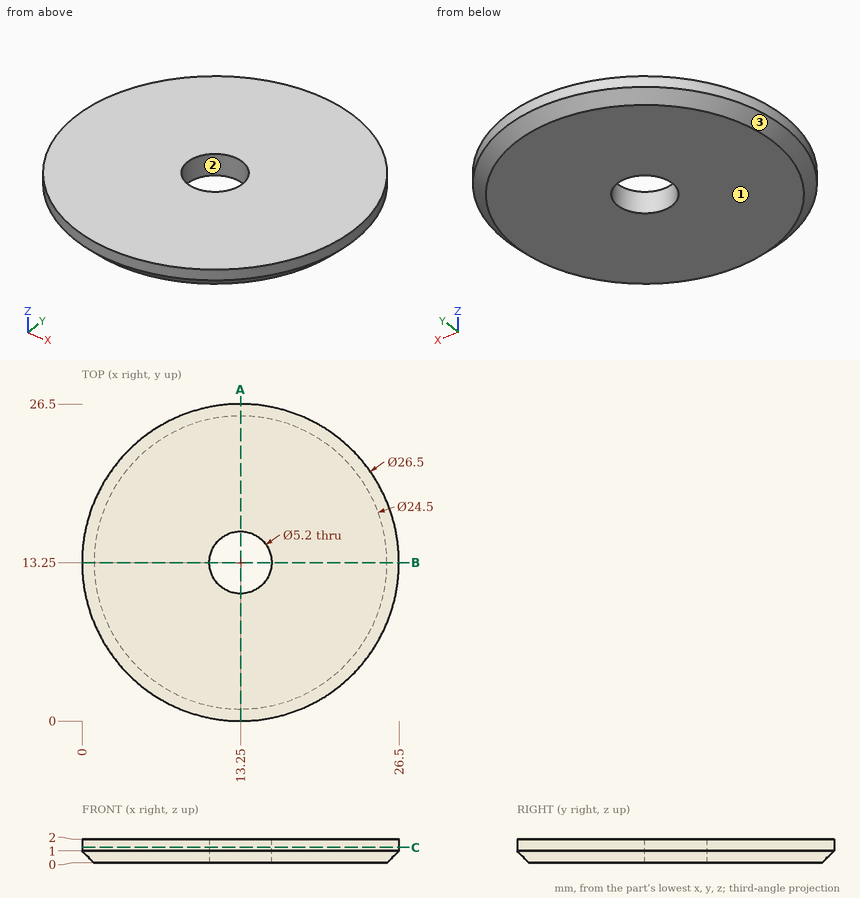
Study the drawing (mm; zero at the part's minimum x, y, z) and answer. Give positions to 0.01 mm unless a question says otherwise; leave off trailing zeros. Order: outer loops, then holes, each group sorted by start corner. A loop starts at its lowest first (then second) coordinate and runs counter-clockwise, first axis right, second up. Notation, with made-up numbers: (-25.75, -11) - (22.25, -11) arc R12 ccw to (22.25, 11) - close; hole circle Ø9 at (25, -4). An arc over 180 degrees is marked (long way). Answer in a Markdown table with one row per item. Add a question column.
Q1. The part is cut by section C-C (z = 1.3). Determine the outline of the cut face in (x, y), then the cut area to 3 significant figures.
Q2. For a pull along X with two mould halves and no side action, classify the marked faces 1, 2 and 3 as released by +X, released by -X, zero draft, split by the parting line, or undercut.
Q3. The part is cut by section A-A (x = 13.25). Determine the outline of the cut face in (y, z), then the cut area to 3 significant figures.
Q4. Find the intervals of material crossed by line 1 along Y through (x, z) = (13.25, 1.25); line 2 along X through (y, z) = (15.25, 1); line 3 along Y through (x, z) = (13.5, 0.6), in increasing order. Write a range as [from, to].
Q5. Given P1, Ø4, axis at x = 13.25, y = 13.25, coming from the +Z side, flat-ended and moving along its own axis, determine where the tip first touches the part or whether it passes through.
Determined:
| question | item | result |
|---|---|---|
| 1 | outline | circle Ø26.5 at (13.25, 13.25); hole circle Ø5.2 at (13.25, 13.25) |
| 1 | area | 530 mm² |
| 2 | face 1 | zero draft |
| 2 | face 2 | undercut |
| 2 | face 3 | split by the parting line |
| 3 | outline | (0, 1) - (1, 0) - (10.65, 0) - (10.65, 2) - (0, 2) - close; (15.85, 0) - (25.5, 0) - (26.5, 1) - (26.5, 2) - (15.85, 2) - close |
| 3 | area | 41.6 mm² |
| 4 | line 1 | y = [0, 10.65], [15.85, 26.5] |
| 4 | line 2 | x = [0.15, 11.59], [14.91, 26.35] |
| 4 | line 3 | y = [0.4, 10.66], [15.84, 26.1] |
| 5 | P1 | passes through |
